Geometry: final body of the model. Coordinates: model frame, mm. Face numbers are marked on the shaded views. A direction names the side the tool comes from. Give positions to 0.01 mm unless a question says otherwise; leave off trailing zeros. Write each loop counter-clockwise with the first axis right and the second up, starting at its lowest first coordinate (ties: lowest second). Pieces come first, ordered by that corner, then holes.
Q1. Section A-A (z = -40). Return the cut outline in (x, y), plus the area to 3 significant figures.
Q2. Section B-B (y = 22). Return the cut outline in (x, z), plus the area to 4 significant figures.
Q3. Section C-C (x = 55). Return the cut outline in (y, z).
Q4. Section D-D (y = 11.5). Return the cut outline in (x, z).
Q5. Line query: line 1 (X direction, y = 1.2, z = 20); line 2 (X direction, y = 9, z = -45.5); line 3 (Y direction, x = 23, z = 24). Output: solid intervals per line, ascending.
Q6. Reachability of the marked faces 4 and 5 from +Z, -Z, +X, -X, +Y, -Y: full face, straight path, thin tool, end or side. Return the list, or none.
Q7. Pin query (flat end, axial travel): pin 1 Ø5 at (y, z) = (5, -37) entering from +X; pin 2 Ø10 at (x, y) = (-9, 10.5) entering from -Z; pin 3 Ø5 at (x, z) = (20.5, -33) entering from -Y; pin 4 Ø1.6 at (x, z) = (44.5, -56.5) entering from -Y. Return the tip coordinate at first contact, or that it passes through.
Q8. Mould query, pull axis X, two halves, no side actions, for the marked faces 1, 2 and 3. Classes: +X half, -X half, draft (parallel to the pull), parting line (faces both ways), or undercut.
from build123d import *

# Parameters (mm, degrees)
SKETCH_1_W          = 115
SKETCH_1_H          = 98.5
EXTRUDE_1_DEPTH     = 35
SKETCH_2_W          = 105
SKETCH_2_H          = 92
CUT_EXTRUDE_1_DEPTH = 33
SKETCH_4_R          = 1.5
CUT_EXTRUDE_2_DEPTH = 3
SKETCH_4_2_R        = 1.5
CUT_EXTRUDE_3_DEPTH = 4
SKETCH_5_W          = 5
SKETCH_5_H          = 70
CUT_EXTRUDE_4_DEPTH = 31
SKETCH_6_R          = 19
CUT_EXTRUDE_5_DEPTH = 2
CUT_EXTRUDE_6_DEPTH = 2
SKETCH_6_3_R        = 19
EXTRUDE_2_DEPTH     = 2
SKETCH_6_5_R        = 19
CUT_EXTRUDE_7_DEPTH = 2


with BuildPart() as part:
    # Sketch 1 → Extrude 1 (new body)
    with BuildSketch(Plane(origin=(0, 0, 0), x_dir=(1, 0, 0), z_dir=(0, 1, 0))):
        with Locations((0, 7.75)):
            Rectangle(SKETCH_1_W, SKETCH_1_H)
    extrude(amount=EXTRUDE_1_DEPTH)

    # Sketch 2 → Cut-Extrude 1 (cut)
    with BuildSketch(Plane.XZ):
        with Locations((0, -9.5)):
            Rectangle(SKETCH_2_W, SKETCH_2_H)
    extrude(amount=-CUT_EXTRUDE_1_DEPTH, mode=Mode.SUBTRACT)

    # Sketch 4 → Cut-Extrude 2 (cut)
    with BuildSketch(Plane(origin=(0, 0, 0), x_dir=(-1, 0, 0), z_dir=(0, -1, 0))):
        with Locations(Location((55, -20, 0), (0, 0, 90))):
            Circle(SKETCH_4_R)
        with Locations(Location((55, 40, 0), (0, 0, 90))):
            Circle(SKETCH_4_R)
        with Locations(Location((-55, -20, 0), (0, 0, 90))):
            Circle(SKETCH_4_R)
        with Locations(Location((-55, 40, 0), (0, 0, 90))):
            Circle(SKETCH_4_R)
    extrude(amount=-CUT_EXTRUDE_2_DEPTH, mode=Mode.SUBTRACT)

    # Sketch 4_2 → Cut-Extrude 3 (cut)
    with BuildSketch(Plane(origin=(0, 0, 0), x_dir=(-1, 0, 0), z_dir=(0, -1, 0))):
        with Locations(Location((55, -20, 0), (0, 0, 90))):
            Circle(SKETCH_4_2_R)
        with Locations(Location((55, 40, 0), (0, 0, 90))):
            Circle(SKETCH_4_2_R)
        with Locations(Location((-55, -20, 0), (0, 0, 90))):
            Circle(SKETCH_4_2_R)
        with Locations(Location((-55, 40, 0), (0, 0, 90))):
            Circle(SKETCH_4_2_R)
    extrude(amount=-CUT_EXTRUDE_3_DEPTH, mode=Mode.SUBTRACT)

    # Sketch 5 → Cut-Extrude 4 (cut)
    with BuildSketch(Plane(origin=(0, 35, 0), x_dir=(1, 0, 0), z_dir=(0, 1, 0))):
        with Locations((-55, 10)):
            Rectangle(SKETCH_5_W, SKETCH_5_H)
        with Locations((55, 10)):
            Rectangle(SKETCH_5_W, SKETCH_5_H)
    extrude(amount=-CUT_EXTRUDE_4_DEPTH, mode=Mode.SUBTRACT)

    # Sketch 6 → Cut-Extrude 5 (cut)
    with BuildSketch(Plane(origin=(0, 35, 0), x_dir=(1, 0, 0), z_dir=(0, 1, 0))):
        with Locations(Location((4, -5, 0), (0, 0, 270))):
            Circle(SKETCH_6_R)
    extrude(amount=-CUT_EXTRUDE_5_DEPTH, mode=Mode.SUBTRACT)

    # Sketch 7 → Cut-Extrude 6 (cut)
    with BuildSketch(Plane(origin=(0, 0, -57), x_dir=(-1, 0, 0), z_dir=(0, 0, -1))):
        Polygon((-50, 0), (50, 0), (50, 10), (36, 10), (36, 20), (-15, 20), (-15, 10), (-35, 10), (-35, 15), (-50, 15), (-50, 10), align=None)
    extrude(amount=-CUT_EXTRUDE_6_DEPTH, mode=Mode.SUBTRACT)

    # Sketch 6_3 → Extrude 2 (add)
    with BuildSketch(Plane(origin=(0, 35, 0), x_dir=(1, 0, 0), z_dir=(0, 1, 0))):
        with Locations((4, -5)):
            Circle(SKETCH_6_3_R)
    extrude(amount=-EXTRUDE_2_DEPTH)

    # Sketch 6_5 → Cut-Extrude 7 (cut)
    with BuildSketch(Plane(origin=(0, 35, 0), x_dir=(1, 0, 0), z_dir=(0, 1, 0))):
        with Locations(Location((4, -5, 0), (0, 0, 270))):
            Circle(SKETCH_6_5_R)
    extrude(amount=-CUT_EXTRUDE_7_DEPTH, mode=Mode.SUBTRACT)


solid = part.part
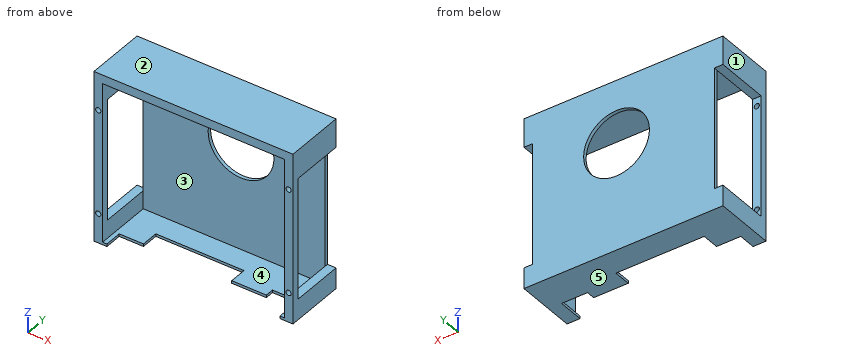
Computed:
1. outline: (-57.5, 0) - (-56.5, 0) - (-56.5, 4) - (-57.5, 4) - close; (-53.5, 0) - (-52.5, 0) - (-52.5, 4) - (-53.5, 4) - close; (-52.5, 33) - (52.5, 33) - (52.5, 35) - (-52.5, 35) - close; (52.5, 0) - (53.5, 0) - (53.5, 4) - (52.5, 4) - close; (56.5, 0) - (57.5, 0) - (57.5, 4) - (56.5, 4) - close
1. area: 226 mm2
2. outline: (-57.5, -57) - (57.5, -57) - (57.5, -45) - (52.5, -45) - (52.5, -55.5) - (-52.5, -55.5) - (-52.5, -45) - (-57.5, -45) - close; (-57.5, 25) - (-52.5, 25) - (-52.5, 36.5) - (52.5, 36.5) - (52.5, 25) - (57.5, 25) - (57.5, 41.5) - (-57.5, 41.5) - close
2. area: 967.5 mm2
3. outline: (0, -57) - (35, -57) - (35, -45) - (4, -45) - (4, -41.5) - (0, -41.5) - close; (0, -38.5) - (4, -38.5) - (4, 18.5) - (0, 18.5) - close; (0, 21.5) - (4, 21.5) - (4, 25) - (35, 25) - (35, 41.5) - (0, 41.5) - close
4. outline: (-57.5, -57) - (-36, -57) - (-36, -55.5) - (-52.5, -55.5) - (-52.5, -45) - (-57.5, -45) - close; (-57.5, 25) - (-52.5, 25) - (-52.5, 36.5) - (52.5, 36.5) - (52.5, 25) - (57.5, 25) - (57.5, 41.5) - (-57.5, 41.5) - close; (15, -57) - (35, -57) - (35, -55.5) - (15, -55.5) - close; (50, -57) - (57.5, -57) - (57.5, -45) - (52.5, -45) - (52.5, -55.5) - (50, -55.5) - close
5. line 1: x = -57.5 to -56.5, -53.5 to -52.5, 52.5 to 53.5, 56.5 to 57.5
5. line 2: x = -57.5 to -52.5, 52.5 to 57.5
5. line 3: y = 33 to 35
6. face 4: -Y
6. face 5: -Z, +X, -X, +Y, -Y
7. pin 1: stops at x = 57.5
7. pin 2: stops at z = 36.5
7. pin 3: stops at y = 33
7. pin 4: stops at y = 15
8. face 1: -X half
8. face 2: draft
8. face 3: undercut
